The drawing under review shows one solid part. Ordinate dimensions are in mm from its lowest x, y, z. A direction names the side the tool comes from. Coordinates: 2 decimals unless noted, no trailing zeros. Loops run counter-clockwise (first coordinate to the right, second up) from the corner with the lowest first, then second, coordinate; pieces in that order, holes last.
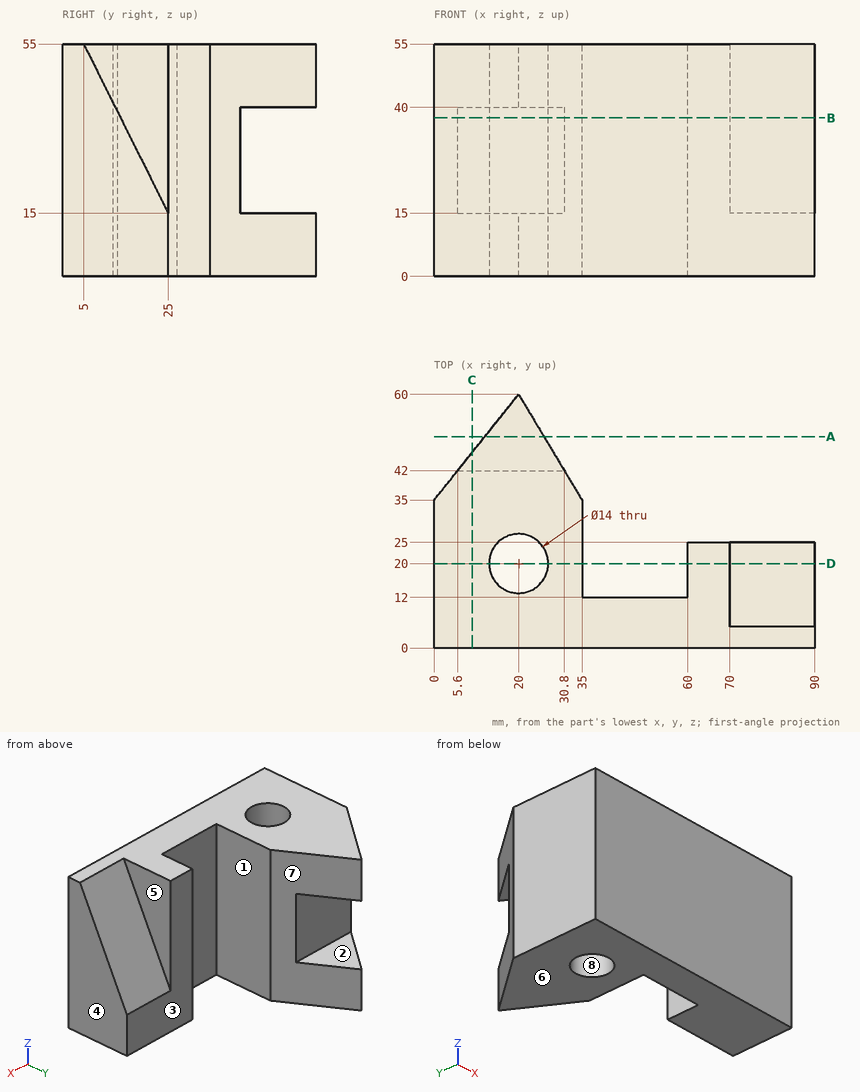
Q1. Machinability: for the marked faces 1, 2, 3, 4 and 5, which of the approach directions +Z, -Z, +X, -X, +Y, -Y give a long, thin tool a straight path to every point of the face, cutting with its end or side? Answer none if there is none.
Q2. Clearance check with flat-ended pins moving along their axes: pin 1 Ø6 at (x, z) = (76.5, 46.5) entering from +Y; pin 2 Ø7.5 at (x, z) = (45.5, 24) entering from +Y; pin 3 Ø15 at (x, z) = (78.5, 29.5) entering from +Y. State where each tip first meets the part, or that it passes through.
Q3. Take a section at B-B, the plane z = 37.5. Write out the cut boundary in (x, y).
Q4. Take a section at A-A, the plane y = 50. Write out the cut boundary in (x, z), then the cut area to 3 significant figures.
Q5. The part is to be moulded in two halves that separate along X. For the marked faces 6, 7 and 8, say which applies: pulls with the +X half, pulls with the -X half, needs draft (parallel to the pull), parting line crosses it, or undercut.
Q6. Take a section at C-C, the plane x = 9. Write out the cut boundary in (y, z), then the cut area to 3 significant figures.
Q7. For line 1 (Y direction, x = 20, z = 39); line 2 (X direction, y = 23, z = 52.5); line 3 (Z direction, x = 18.5, y = 56.5), list the stretches that pass through material, from the lowest coordinate up.
Q8. Take a section at D-D, the plane y = 20. Write out the cut boundary in (x, z), then the cut area to 4 significant figures.
Entries:
1. face 1: +Z, -Z, +Y
1. face 2: +X, -X, +Y
1. face 3: +Z, -Z, +X, +Y
1. face 4: +Z, -Z, +X, +Y, -Y
1. face 5: +Z, +X, +Y
2. pin 1: stops at y = 10.75
2. pin 2: stops at y = 12
2. pin 3: stops at y = 21.5
3. outline: (0, 0) - (90, 0) - (90, 13.75) - (70, 13.75) - (70, 25) - (60, 25) - (60, 12) - (35, 12) - (35, 35) - (30.8, 42) - (5.6, 42) - (0, 35) - close; hole circle Ø14 at (20, 20)
4. outline: (12, 0) - (26, 0) - (26, 15) - (12, 15) - close; (12, 40) - (26, 40) - (26, 55) - (12, 55) - close
4. area: 420 mm2
5. face 6: needs draft
5. face 7: pulls with the +X half
5. face 8: undercut
6. outline: (0, 0) - (46.25, 0) - (46.25, 15) - (42, 15) - (42, 40) - (46.25, 40) - (46.25, 55) - (0, 55) - close
6. area: 2,440 mm2
7. line 1: y = 0 to 13, 27 to 42
7. line 2: x = 0 to 13.68, 26.32 to 35, 60 to 70
7. line 3: z = 0 to 15, 40 to 55
8. outline: (0, 0) - (13, 0) - (13, 55) - (0, 55) - close; (27, 0) - (35, 0) - (35, 55) - (27, 55) - close; (60, 0) - (90, 0) - (90, 25) - (70, 25) - (70, 55) - (60, 55) - close
8. area: 2,205 mm2
